Build history of the part. All positions in model axes, mm. A direction names the side the tool comes from. Round coordinates to 2 decimals unless told otherwise and drop trailing zeros. Loops run counter-clockwise (first coordinate to the right, second up) from the corner with the lowest first, then second, coordinate; pieces in that order, holes last. Notation, with made-up numbers: (4.5, -10) - (56.5, -10) arc R24 cw to (56.5, 6) - close; hole circle Ø5 at (46, 49.5). An arc over 180 degrees is marked (long way). Use a Markdown table: item, result.
from build123d import *

# Parameters (mm, degrees)
CROQUIS1_W              = 1920
CROQUIS1_H              = 2100
SALIENTE_EXTRUIR1_DEPTH = 10
CROQUIS2_W              = 1920
CROQUIS2_H              = 1980
CORTAR_EXTRUIR1_DEPTH   = 3
CROQUIS3_W              = 1920
CROQUIS3_H              = 1980
CORTAR_EXTRUIR2_DEPTH   = 3
CROQUIS4_W              = 10
CROQUIS4_H              = 1980
CORTAR_EXTRUIR3_DEPTH   = 8
MATRIZL1_COUNT          = 8
MATRIZL1_PITCH          = 210
CROQUIS5_W              = 200
CROQUIS5_H              = 1980
CORTAR_EXTRUIR4_DEPTH   = 10


with BuildPart() as part:
    # Croquis1 → Saliente-Extruir1 (new body)
    with BuildSketch(Plane.XY):
        with Locations((960, -1050)):
            Rectangle(CROQUIS1_W, CROQUIS1_H)
    extrude(amount=SALIENTE_EXTRUIR1_DEPTH)

    # Croquis2 → Cortar-Extruir1 (cut)
    with BuildSketch(Plane.XY.offset(10)):
        with Locations((960, -1110)):
            Rectangle(CROQUIS2_W, CROQUIS2_H)
    extrude(amount=-CORTAR_EXTRUIR1_DEPTH, mode=Mode.SUBTRACT)

    # Croquis3 → Cortar-Extruir2 (cut)
    with BuildSketch(Plane(origin=(0, 0, 0), x_dir=(-1, 0, 0), z_dir=(0, 0, -1))):
        with Locations((-960, -1110)):
            Rectangle(CROQUIS3_W, CROQUIS3_H)
    extrude(amount=-CORTAR_EXTRUIR2_DEPTH, mode=Mode.SUBTRACT)

    # Croquis4 → Cortar-Extruir3 (cut)
    with BuildSketch(Plane(origin=(0, 0, 3), x_dir=(-1, 0, 0), z_dir=(0, 0, -1))):
        with Locations((-1715, -1110)):
            Rectangle(CROQUIS4_W, CROQUIS4_H)
    cortar_extruir3 = extrude(amount=-CORTAR_EXTRUIR3_DEPTH, mode=Mode.SUBTRACT)

    # MatrizL1: Cortar-Extruir3 ×8
    with Locations(*[(-i * MATRIZL1_PITCH, 0, 0) for i in range(1, MATRIZL1_COUNT)]):
        add(cortar_extruir3, mode=Mode.SUBTRACT)

    # Croquis5 → Cortar-Extruir4 (cut)
    with BuildSketch(Plane(origin=(0, 0, 3), x_dir=(-1, 0, 0), z_dir=(0, 0, -1))):
        with Locations((-980, -1110)):
            Rectangle(CROQUIS5_W, CROQUIS5_H)
    extrude(amount=-CORTAR_EXTRUIR4_DEPTH, mode=Mode.SUBTRACT)


solid = part.part
Q1. Cut at B-B, the plane x = 1544. List the corners of the cut face in (y, z).
Results found:
| item | result |
|---|---|
| outline | (-2100, 3) - (-120, 3) - (-120, 0) - (0, 0) - (0, 10) - (-120, 10) - (-120, 7) - (-2100, 7) - close |
Q2. Cut at C-C, the plane z = 1.5. List the corners of the cut face in (x, y).
Results found:
| item | result |
|---|---|
| outline | (0, -120) - (1920, -120) - (1920, 0) - (0, 0) - close |
Q3. Drop flat-ended pins along their axis: pin 1 (3 mm diameter, centred on x = 981, z = 5, fed in from -Y); pin 2 (12 mm diameter, centred on x = 802, y = -240.5, fed in from -Z). Give the stop position or say it passes through.
Results found:
| item | result |
|---|---|
| pin 1 | stops at y = -120 |
| pin 2 | stops at z = 3 |
Q4. Cut at D-D, the plane x = 908. List the corners of the cut face in (y, z).
Results found:
| item | result |
|---|---|
| outline | (-120, 0) - (0, 0) - (0, 10) - (-120, 10) - close |
Q5. Probe line 1 (Y direction, x = 513.5, z = 0.75); line 2 (Z direction, x = 413, y = -179.5). List the from-to ranges inside material, lowest first.
Results found:
| item | result |
|---|---|
| line 1 | y = -120 to 0 |
| line 2 | z = 3 to 7 |
Q6. Which spindle directions (+Z, -Z, +X, -X, +Y, -Y) get a long thin tool onto all of the face, cutting with end or side? Do faces 1 (the face through (561, -1096, 3)), 2 (the face through (947, -59, 0)), 3 (the face through (1189, -1096, 7)). Say none if no direction does.
Results found:
| item | result |
|---|---|
| face 1 | -Z, +X, -X, -Y |
| face 2 | -Z, +X, -X, +Y, -Y |
| face 3 | +Z, +X, -X, -Y |
Q7. Cut at A-A, the plane y = -1596. Count the separate pieces of the cut face and the enclosed holes in it, plus the area to 3 significant figures.
Results found:
| item | result |
|---|---|
| separate pieces | 8 |
| enclosed holes | 0 |
| area | 6,560 mm2 |
